```python
from build123d import *

# Parameters (mm, degrees)
SKETCH1_R           = 6
SKETCH1_R_2         = 1.5
BOSS_EXTRUDE1_DEPTH = 5
CUT_EXTRUDE1_DEPTH  = 3
SKETCH7_W           = 1
SKETCH7_H           = 7.146818719
CUT_EXTRUDE2_DEPTH  = 10
CIRPATTERN1_COUNT   = 12


with BuildPart() as part:
    # Sketch1 → Boss-Extrude1 (new body)
    with BuildSketch(Plane(origin=(0, 0, 0), x_dir=(1, 0, 0), z_dir=(0, 1, 0))):
        Circle(SKETCH1_R)
        Circle(SKETCH1_R_2, mode=Mode.SUBTRACT)
    extrude(amount=BOSS_EXTRUDE1_DEPTH)

    # Sketch6 → Cut-Extrude1 (cut)
    with BuildSketch(Plane(origin=(0, 5, 0), x_dir=(1, 0, 0), z_dir=(0, 1, 0))):
        Polygon((2.825, -1.63101451), (2.825, 1.63101451), (0, 3.262029021), (-2.825, 1.63101451), (-2.825, -1.63101451), (0, -3.262029021), align=None)
    extrude(amount=-CUT_EXTRUDE1_DEPTH, mode=Mode.SUBTRACT)

    # Sketch7 → Cut-Extrude2 (cut)
    with BuildSketch(Plane(origin=(0, 5, 0), x_dir=(1, 0, 0), z_dir=(0, 1, 0))):
        with Locations((0, 8.37340936)):
            Rectangle(SKETCH7_W, SKETCH7_H)
    cut_extrude2 = extrude(amount=-CUT_EXTRUDE2_DEPTH, mode=Mode.SUBTRACT)

    # CirPattern1: Cut-Extrude2 ×12 about axis
    cirpattern1_axis = Axis((0, 0, 0), (0, 1, 0))
    for i in range(1, CIRPATTERN1_COUNT):
        add(cut_extrude2.rotate(cirpattern1_axis, i * 360 / CIRPATTERN1_COUNT), mode=Mode.SUBTRACT)


solid = part.part
```
The model under review builds one solid part; all positions refer to its coordinate system, in mm. A direction names the side the tool comes from. Give positions to 0.01 mm unless a question says otherwise; leave off trailing zeros. Write each loop counter-clockwise with the first axis right and the second up, starting at its lowest first coordinate (ties: lowest second). Pieces come first, ordered by that corner, then holes. Notation, with made-up numbers: M 6.5,61 L 48.5,61 A29 cw 48.5,88 Z; hole C -38.5,12 d7. An arc over 180 degrees is marked long. Write each question's results on one line, items separated by ' | '. Start each with the question number.
1. For faces 1 (the flat face through (-2.258, 2.535, -4.91)), 2 (the flat face through (0.5, 3, 5)), 3 (the flat face through (5, 3, -0.5)), 4 (the flat face through (1.39, 3.52, 2.46)), list the 3-axis set-ups (+Z, -Z, +X, -X, +Y, -Y) from which the entire face can be reached by the end or side of a thin tool; tool diameter is ignored.
2. We need section A-A (z = 0). Write out the cut boundary in (x, y) (3 decimals).
3. Mouldability with a two-part tool opening along X and no side actions: class faces 5 (the cylindrical face through (4.253, 2.465, -4.232)), 6 (the flat face through (4.15, 2.54, -2.41)), 7 (the flat face through (2.394, 2.535, -4.16)), 8 (the cylindrical face through (-5.79, 2.46, -1.57)) as released by +X, released by -X, zero draft, split by the parting line, or undercut.
4. For probe 1 along X at (y, z) = (1.05, 0); probe 2 along Z at (x, y) = (-4, 4.55), list the stretches that pass through material, from the lowest coordinate up. Write a range as [from, to].
5. Insertion check: pin 1 Ø1.3 at (y, z) = (3, 5.5) entering from +X; pin 2 Ø6 at (x, z) = (2.5, -1.5) entering from +Y; pin 3 Ø0.8 at (y, z) = (3, 0) entering from -X; pin 4 Ø0.6 at (x, y) = (5.5, 1.5) entering from +Z. Each pin has a flat end and moves straight along its axis. Give the tip position at first contact, or say it passes through.
6. We need section B-B (x = 3.25). Write out the cut boundary in (y, z).
Results found:
1) face 1: +Y, -Y | face 2: +Z, +Y, -Y | face 3: +X, +Y, -Y | face 4: +Y
2) outline: M -4.8,0 L -1.5,0 L -1.5,2 L -2.825,2 L -2.825,5 L -4.8,5 Z; M 1.5,0 L 4.8,0 L 4.8,5 L 2.825,5 L 2.825,2 L 1.5,2 Z
3) face 5: released by +X | face 6: undercut | face 7: undercut | face 8: released by -X
4) probe 1: x = [-4.8, -1.5], [1.5, 4.8] | probe 2: z = [-4.47, -2.89], [-2.67, 2.67], [2.89, 4.47]
5) pin 1: stops at x = 3.53 | pin 2: stops at y = 5 | pin 3: stops at x = -4.8 | pin 4: stops at z = 2.56
6) outline: M 0,-4.63 L 5,-4.63 L 5,4.63 L 0,4.63 Z
